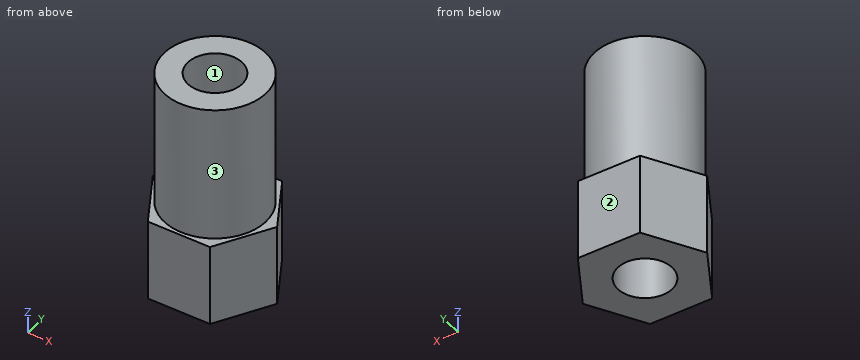
from build123d import *

# Parameters (mm, degrees)
F1_DEPTH = 6
F2_R     = 3.75
F3_DEPTH = 10
F4_R     = 2
F5_DEPTH = 25


with BuildPart() as f1:
    # F0 (on Top) → F1 (new body)
    with BuildSketch(Plane.XY):
        Polygon((-17.257317, 9.717025), (-21.87612, 9.717025), (-24.185521, 5.717025), (-21.87612, 1.717025), (-17.257317, 1.717025), (-14.947916, 5.717025), align=None)
    extrude(amount=F1_DEPTH)

    # F2 (on face) → F3 (join)
    with BuildSketch(Plane.XY.offset(6)):
        with Locations((-19.566718, 5.717025)):
            Circle(F2_R)
    extrude(amount=F3_DEPTH)

    # F4 (on face) → F5 (cut)
    with BuildSketch(Plane(origin=(0, 0, 0), x_dir=(1, 0, 0), z_dir=(0, 0, -1))):
        with Locations((-19.566718, -5.717025)):
            Circle(F4_R)
    extrude(amount=-F5_DEPTH, mode=Mode.SUBTRACT)


solid = f1.part
Could you check a few things on this model? Use its own coordinates, in mm. Face numbers are marked on the shaded views. Give positions to 0.01 mm unless a question says otherwise; leave off trailing zeros. Order: outer loops, then holes, each group sorted by start corner. A loop starts at its lowest first (then second) coordinate and runs counter-clockwise, first axis right, second up.
1. Thinking about a two-plate mould opening in X: for the marked faces 1, 2 and 3, which applies, +X half, -X half, draft (parallel to the pull), parting line (faces both ways), or undercut?
Answers below:
face 1: undercut
face 2: draft
face 3: parting line
2. Suppose I cut it at B-B (y = 7.5). Write out the boundary of the cut face in (x, z).
Answers below:
outline: (-23.16, 0) - (-20.47, 0) - (-20.47, 16) - (-22.87, 16) - (-22.87, 6) - (-23.16, 6) - close; (-18.66, 0) - (-15.98, 0) - (-15.98, 6) - (-16.27, 6) - (-16.27, 16) - (-18.66, 16) - close
3. Suppose I cut it at C-C (x = -18.5). Write out the boundary of the cut face in (y, z).
Answers below:
outline: (1.72, 0) - (4.03, 0) - (4.03, 16) - (2.12, 16) - (2.12, 6) - (1.72, 6) - close; (7.41, 0) - (9.72, 0) - (9.72, 6) - (9.31, 6) - (9.31, 16) - (7.41, 16) - close
4. I need wall thicknesses on L1, parallel to X at y = 6.75, z = 1.25; L2, parallel to X at y = 5, z = 8.25; L3, parallel to Y at x = -20.25, z = 1. Which ranges of each line are inside material? Lowest first, please.
Answers below:
L1: x = -23.59 to -21.28, -17.85 to -15.54
L2: x = -23.25 to -21.43, -17.7 to -15.89
L3: y = 1.72 to 3.84, 7.6 to 9.72
5. Suppose I cut it at D-D (x = -16.5). Write out the boundary of the cut face in (y, z), plus the area to 3 significant figures.
Answers below:
outline: (3.03, 0) - (8.41, 0) - (8.41, 6) - (7.88, 6) - (7.88, 16) - (3.56, 16) - (3.56, 6) - (3.03, 6) - close
area: 75.4 mm2
6. Suppose I cut it at A-A (z = 2.75). Write out the boundary of the cut face in (x, y), plus the area to 3 significant figures.
Answers below:
outline: (-24.19, 5.72) - (-21.88, 1.72) - (-17.26, 1.72) - (-14.95, 5.72) - (-17.26, 9.72) - (-21.88, 9.72) - close; hole circle Ø4 at (-19.57, 5.72)
area: 42.9 mm2
